Source: CAD feature listing. Evaluate the final solid. Frame: model axes, mm. A direction names the side the tool comes from. Round coordinates to 2 decimals unless told otherwise and drop trailing zeros. Write each loop counter-clockwise with the first axis right and the second up, starting at its lowest first coordinate (ties: lowest second). Pieces come first, ordered by that corner, then holes. Notation, with made-up numbers: M 69.5,38 L 105.5,38 A26 ccw 105.5,59 Z; hole C 85.25,-7.75 d4. An arc over 180 degrees is marked long. Answer in a Markdown table with one row per item.
from build123d import *

# Parameters (mm, degrees)
F0_W     = 3
F0_H     = 40
F1_DEPTH = 16
F3_D     = 6
F4_W     = 40
F4_H     = 3
F5_DEPTH = 4
F7_DEPTH = 25


with BuildPart() as f1:
    # F0 (on Top) → F1 (new body)
    with BuildSketch(Plane.XY):
        Polygon((-1.5, 23), (-1.5, 20), (1.5, 20), (10.5, 20), (10.5, 23), align=None)
        Rectangle(F0_W, F0_H)
        Polygon((1.5, -20), (-1.5, -20), (-1.5, -23), (10.5, -23), (10.5, -20), align=None)
    extrude(amount=F1_DEPTH)

    # F3 (through all)
    with Locations(Plane.XZ.offset(23)):
        with Locations((4.5, 12)):
            Hole(F3_D / 2)

    # F4 (on face) → F5 (join)
    with BuildSketch(Plane.YZ.offset(1.5)):
        with Locations((0, 1.5)):
            Rectangle(F4_W, F4_H)
    extrude(amount=F5_DEPTH)

    # F6 (on face) → F7 (cut)
    with BuildSketch(Plane.YZ.offset(1.5)):
        Polygon((20, 16), (-20, 16), (-20, 12), (-20, 3), (20, 3), (20, 12), align=None)
    extrude(amount=-F7_DEPTH, mode=Mode.SUBTRACT)


solid = f1.part
Q1. Contact query for flat-ended pins moving along their axis: pin 1 Ø2 at (y, z) = (2, 5.5) entering from -X; pin 2 Ø0.9 at (y, z) = (2.5, 1) entering from +X. Output: stop coordinate, or through.
Solutions:
| item | result |
|---|---|
| pin 1 | passes through |
| pin 2 | stops at x = 5.5 |
Q2. Section A-A (x = 4.5). Return loops of the section in (y, z).
Solutions:
| item | result |
|---|---|
| outline | M -23,0 L 23,0 L 23,9 L 20,9 L 20,3 L -20,3 L -20,9 L -23,9 Z; M -23,15 L -20,15 L -20,16 L -23,16 Z; M 20,15 L 23,15 L 23,16 L 20,16 Z |
Q3. Section C-C (z = 12). Return loops of the section in (x, y), and give its area (3 significant figures).
Solutions:
| item | result |
|---|---|
| outline | M -1.5,-23 L 1.5,-23 L 1.5,-20 L -1.5,-20 Z; M -1.5,20 L 1.5,20 L 1.5,23 L -1.5,23 Z; M 7.5,-23 L 10.5,-23 L 10.5,-20 L 7.5,-20 Z; M 7.5,20 L 10.5,20 L 10.5,23 L 7.5,23 Z |
| area | 36.0 mm2 |
Q4. Material intervals for probe 1 along Z at (x, y) = (4.5, 22.2); probe 2 along Y at (x, z) = (-0.25, 13); probe 3 along Z at (x, y) = (5, 11), sorted ascending.
Solutions:
| item | result |
|---|---|
| probe 1 | z = 0 to 9, 15 to 16 |
| probe 2 | y = -23 to -20, 20 to 23 |
| probe 3 | z = 0 to 3 |
Q5. Section B-B (z = 8). Return loops of the section in (x, y).
Solutions:
| item | result |
|---|---|
| outline | M -1.5,-23 L 10.5,-23 L 10.5,-20 L -1.5,-20 Z; M -1.5,20 L 10.5,20 L 10.5,23 L -1.5,23 Z |
Q6. Pull-direction query (X, two-part tool) for faces 5 (the flat face through (10.5, -22, 8)), 6 (the flat face through (3, 0, 0)), 7 (the cylindrical face through (1.64, -21.48, 12.9)); classes: pulls with the +X half, pulls with the -X half, needs draft (parallel to the pull), parting line crosses it, or undercut.
Solutions:
| item | result |
|---|---|
| face 5 | pulls with the +X half |
| face 6 | needs draft |
| face 7 | undercut |
Q7. Access query for faces 1 (the flat face through (5.5, 0, 2)), 2 (the flat face through (-1.5, 0.3, 2.6)), 3 (the flat face through (2, 0, 3)), 4 (the flat face through (4, 20, 8)). Directions: +Z, -Z, +X, -X, +Y, -Y. A direction counts if a zero-diameter tool reaches every point of the face in a straight line with its end or side. Return the directions, or none.
Solutions:
| item | result |
|---|---|
| face 1 | +Z, -Z, +X |
| face 2 | +Z, -Z, -X, +Y, -Y |
| face 3 | +Z, +X, -X |
| face 4 | +Z, +X |
Q8. Section D-D (x = 6.5). Return loops of the section in (y, z), and give its area (3 significant figures).
Solutions:
| item | result |
|---|---|
| outline | M -23,0 L -20,0 L -20,9.76 L -23,9.76 Z; M -23,14.24 L -20,14.24 L -20,16 L -23,16 Z; M 20,0 L 23,0 L 23,9.76 L 20,9.76 Z; M 20,14.24 L 23,14.24 L 23,16 L 20,16 Z |
| area | 69.2 mm2 |
